from build123d import *

# Parameters (mm, degrees)
F2_R     = 12.5
F3_DEPTH = 100
F4_R     = 35.5
F5_DEPTH = 29
F6_R     = 31.8
F7_DEPTH = 8


with BuildPart() as f1:
    # F0 (on Right) → F1 (revolve)
    with BuildSketch(Plane.YZ):
        Polygon((0, 0), (0, 15), (-35.5, 10), (-35.5, 0), align=None)
    revolve(axis=Axis((0, 0, 2.476192), (0, 0, 1)))

    # F2 (on Top) → F3 (join)
    with BuildSketch(Plane.XY):
        Circle(F2_R)
    extrude(amount=F3_DEPTH)

    # F4 (on face) → F5 (join)
    with BuildSketch(Plane.XY.offset(100)):
        Circle(F4_R)
    extrude(amount=F5_DEPTH)

    # F6 (on face) → F7 (join)
    with BuildSketch(Plane.XY.offset(129)):
        Circle(F6_R)
    extrude(amount=F7_DEPTH)


solid = f1.part
CAD build for the part. Positions are in the model's coordinates, mm. A direction names the side the tool comes from. Give positions to 0.01 mm unless a question says otherwise; leave off trailing zeros. Write each loop counter-clockwise with the first axis right and the second up, starting at its lowest first coordinate (ties: lowest second). Pieces come first, ordered by that corner, then holes. Notation, with made-up numbers: (47.25, 89.5) -> (53.25, 89.5) arc R28 cw to (53.25, 115.5) -> close; hole circle Ø2 at (75, -2.5). An arc over 180 degrees is marked (long way). Return JSON: item names as keys, results as strings.
Item 1: Tool access for faces 1 (the flat face through (0, -15, 100)), 2 (the cylindrical face through (-34.656, 7.696, 4.93)), 3 (the cylindrical face through (-6.894, -31.044, 132.944)): list every direction of +Z, -Z, +X, -X, +Y, -Y with a clear straight run to the whole face (end or side of a thin tool).
Answer below:
{"face 1": "none", "face 2": "+Z, -Z", "face 3": "+Z"}
Item 2: Two-plate mould, pull along Z, no slides. Class faces 4 (the flat face through (0, 0, 137)), 5 (the cylindrical face through (-7.696, -34.656, 114.297)), 6 (the cylindrical face through (11.923, 3.755, 56.012)): +Z half, -Z half, draft (parallel to the pull), parting line (faces both ways), or undercut.
Answer below:
{"face 4": "+Z half", "face 5": "draft", "face 6": "undercut"}
Item 3: Drop a flat-ended pin along its axis: pin 1 (2 mm diameter, centred on x = 3.5, z = 46.5, fed in from +Y). Give the stop position or say it passes through.
Answer below:
{"pin 1": "stops at y = 12.25"}
Item 4: Band-saw the part on A-A (x = 0). List the corners of the cut face in (y, z).
Answer below:
{"outline": "(-35.5, 0) -> (35.5, 0) -> (35.5, 10) -> (12.5, 13.24) -> (12.5, 100) -> (35.5, 100) -> (35.5, 129) -> (31.8, 129) -> (31.8, 137) -> (-31.8, 137) -> (-31.8, 129) -> (-35.5, 129) -> (-35.5, 100) -> (-12.5, 100) -> (-12.5, 13.24) -> (-35.5, 10) -> close"}
Item 5: Drill centre lines: probe 1 along Z at (x, y) = (-8, -16); probe 2 along Z at (x, y) = (-30, 14.5); probe 3 along Y at (x, z) = (2.5, 55.5). Where is each one in solid material? Low to high.
Answer below:
{"probe 1": "z = 0 to 12.48, 100 to 137", "probe 2": "z = 0 to 10.31, 100 to 129", "probe 3": "y = -12.25 to 12.25"}
Item 6: Band-saw the part on C-C (z = 76.5). List the corners of the cut face in (x, y).
Answer below:
{"outline": "circle Ø25 at (0, 0)"}
